Autodesk Inventor part; units mm, degrees
ref_plane "YZ Plane" through (0, 0, 0) normal (1, 0, 0) x (0, 1, 0)
ref_plane "XZ Plane" through (0, 0, 0) normal (0, 1, 0) x (-1, 0, 0)
ref_plane "XY Plane" through (0, 0, 0) normal (0, 0, 1) x (1, 0, 0)
sketch "Sketch1" plane through (0, 0, 0) normal (0, 0, 1) x (1, 0, 0)
  line L0 (-30, 40) -> (0, 40)
  line L1 (-36.1318, 34) -> (13.8682, 34) construction
  arc A0 (0, 30) -> (0, 38) centre (0, 34) ccw
  arc A1 (-30, 30) -> (-30, 38) centre (-30, 34) ccw
  line L2 (-30, 30) -> (0, 30) construction
  line L3 (-30, 0) -> (-30, -4.5) construction
  line L4 (-30, -4.5) -> (0, -4.5) construction
  line L5 (0, -4.5) -> (0, 0) construction
  circle A2 centre (-30, -4.5) radius 4 construction
  circle A3 centre (0, -4.5) radius 4 construction
  line L6 (-30, 0) -> (-30, 30)
  line L7 (-30, 38) -> (-30, 40)
  line L8 (0, 40) -> (0, 38)
  line L9 (0, 30) -> (0, 0)
  line L10 (-30, 0.0688) -> (-30, -0.5)
  line L11 (-30, -0.5) -> (-26, -4.5)
  line L12 (0, 0) -> (0, -0.5)
  line L13 (0, -0.5) -> (4, -4.5)
  line L14 (4, -4.5) -> (0, -8.5)
  line L15 (-26, -4.5) -> (-30, -8.5)
  line L16 (-30, -8.5) -> (-30, -10.5)
  line L17 (-30, -10.5) -> (0, -10.5)
  line L18 (0, -10.5) -> (0, -8.5)
  line L19 (0, 0) -> (-0.5, 0)
  dimension "d0" = 30
  dimension "d1" = 40
  dimension "d2" = 50
  dimension "d3" = 6
  dimension "d4" = 8
  dimension "d5" = 8
  dimension "d6" = 4.5
  dimension "d7" = 8
  dimension "d8" = 8
  dimension "d9" = 2
extrude "Extrusion1" add sketch "Sketch1" along normal blind 3
sketch "Sketch2" plane through (0, 0, 3) normal (0, 0, 1) x (1, 0, 0)
  line L0 (-30, -10.5) -> (0, -10.5) construction
  line L1 (0, -0.5) -> (0, 30) construction
  line L2 (0, 40) -> (-30, 40) construction
  line L3 (-15, 40) -> (-15, -10.5) construction
  line L4 (-15, 40) -> (-15, 36.5) construction
  line L5 (-15, 36.5) -> (-8.9843, 36.5) construction
  line L6 (-17.7725, 36.2895) -> (-9.6231, 36.2895) construction
  line L7 (-9.6231, 36.2895) -> (-9.6231, 27.3992) construction
  line L8 (-9.6231, 27.3992) -> (-17.7725, 27.3992) construction
  line L9 (-17.7725, 27.3992) -> (-17.7725, 36.2895) construction
  line L10 (-15, -10.5) -> (-15, 26) construction
  line L11 (-15, 26) -> (0, 26) construction
  line L12 (-5.7398, 26) -> (-28, 26)
  line L13 (-28, 26) -> (-28, 24)
  line L14 (-28, 24) -> (-5.7398, 24)
  line L15 (-5.7398, 24) -> (-5.7398, 26)
  line L16 (-28, 25) -> (0, 25) construction
  line L17 (-5.7398, 26) -> (-5.7398, 27.5)
  line L18 (-5.7398, 27.5) -> (-1.4096, 25)
  line L19 (-5.7398, 24) -> (-5.7398, 22.5)
  line L20 (-5.7398, 22.5) -> (-1.4096, 25)
  spline S0 degree 2 poles (-14.5989, 29.9621) (-15.2464, 29.9621) (-16.3191, 30.3575) (-16.7047, 30.7579) knots 0 0 0 1 2 2 2
  spline S1 degree 2 poles (-16.7047, 30.7579) (-17.0903, 31.1633) (-17.5006, 32.3596) (-17.5006, 33.1357) knots 0 0 0 1 2 2 2
  spline S2 degree 2 poles (-17.5006, 33.1357) (-17.5006, 33.8722) (-17.0853, 35.0388) (-16.6998, 35.4541) knots 0 0 0 1 2 2 2
  spline S3 degree 2 poles (-16.6998, 35.4541) (-16.329, 35.8545) (-15.2415, 36.2895) (-14.5939, 36.2895) knots 0 0 0 1 2 2 2
  spline S4 degree 2 poles (-14.5939, 36.2895) (-14.2825, 36.2895) (-13.719, 36.2005) (-13.4619, 36.1214) knots 0 0 0 1 2 2 2
  spline S5 degree 2 poles (-13.4619, 36.1214) (-13.2543, 36.0621) (-12.7501, 35.8446) (-12.5969, 35.7655) knots 0 0 0 1 2 2 2
  line L21 (-12.5969, 35.7655) -> (-12.5969, 34.7867)
  line L22 (-12.5969, 34.7867) -> (-12.6661, 34.7867)
  spline S6 degree 2 poles (-12.6661, 34.7867) (-12.8193, 34.9202) (-13.1406, 35.1624) (-13.4372, 35.3008) knots 0 0 0 1 2 2 2
  spline S7 degree 2 poles (-13.4372, 35.3008) (-13.6844, 35.4244) (-14.3221, 35.5875) (-14.6879, 35.5875) knots 0 0 0 1 2 2 2
  spline S8 degree 2 poles (-14.6879, 35.5875) (-15.5678, 35.5875) (-16.6553, 34.2627) (-16.6553, 33.1604) knots 0 0 0 1 2 2 2
  spline S9 degree 2 poles (-16.6553, 33.1604) (-16.6553, 32.5474) (-16.3686, 31.628) (-16.0967, 31.3116) knots 0 0 0 1 2 2 2
  spline S10 degree 2 poles (-16.0967, 31.3116) (-15.8347, 30.9952) (-15.0932, 30.664) (-14.6285, 30.664) knots 0 0 0 1 2 2 2
  spline S11 degree 2 poles (-14.6285, 30.664) (-14.2875, 30.664) (-13.6053, 30.7629) (-13.3729, 30.8618) knots 0 0 0 1 2 2 2
  line L23 (-13.3729, 30.8618) -> (-13.3729, 32.4387)
  line L24 (-13.3729, 32.4387) -> (-14.7867, 32.4387)
  line L25 (-14.7867, 32.4387) -> (-14.7867, 33.1505)
  line L26 (-14.7867, 33.1505) -> (-12.5721, 33.1505)
  line L27 (-12.5721, 33.1505) -> (-12.5721, 30.4861)
  spline S12 degree 2 poles (-12.5721, 30.4861) (-12.7254, 30.4169) (-13.2494, 30.2043) (-13.4718, 30.14) knots 0 0 0 1 2 2 2
  spline S13 degree 2 poles (-13.4718, 30.14) (-13.7734, 30.0511) (-14.2578, 29.9621) (-14.5989, 29.9621) knots 0 0 0 1 2 2 2
  point P0 (0, 0)
  dimension "d12" = 3.5
  dimension "d13" = 36.5
  dimension "d14" = 2
  dimension "d15" = 1.5
  dimension "d16" = 5
  dimension "d17" = 1.5
  dimension "d58" = 14
extrude "Extrusion2" cut sketch "Sketch2" against normal blind 1
sketch "Sketch5" plane through (0, 0, 0) normal (0, 0, -1) x (-1, 0, 0)
  line L0 (30, 30) -> (30, -0.5) construction
  arc A0 (30, 38) -> (30, 30) centre (30, 34) ccw construction
  line L1 (30, 40) -> (30, 38) construction
  line L2 (0, 40) -> (30, 40) construction
  line L3 (0, 38) -> (0, 40) construction
  arc A1 (0, 38) -> (0, 30) centre (0, 34) ccw construction
  line L4 (0, -0.5) -> (0, 30) construction
  line L5 (-4, -4.5) -> (0, -0.5) construction
  line L6 (0, -8.5) -> (-4, -4.5) construction
  line L7 (0, -10.5) -> (0, -8.5) construction
  line L8 (30, -10.5) -> (0, -10.5) construction
  line L9 (30, -8.5) -> (30, -10.5) construction
  line L10 (26, -4.5) -> (30, -8.5) construction
  line L11 (30, -0.5) -> (26, -4.5) construction
  point P0 (0, 0)
sketch "Sketch6" plane through (0, 0, 0) normal (0, 0, -1) x (-1, 0, 0)
  line L0 (30, 30) -> (30, -0.5) construction
  line L1 (0, 40) -> (30, 40) construction
  line L2 (30, -10.5) -> (0, -10.5) construction
  line L3 (17.9728, -6.9957) -> (10.1851, -6.9957) construction
  line L4 (10.1851, -6.9957) -> (10.1851, 2.1518) construction
  line L5 (10.1851, 2.1518) -> (17.9728, 2.1518) construction
  line L6 (17.9728, 2.1518) -> (17.9728, -6.9957) construction
  line L7 (15, -10.5) -> (15, 40) construction
  line L8 (15, -10.5) -> (15, -7) construction
  line L9 (15, -7) -> (11.2598, -7) construction
  line L10 (16.564, 40) -> (16.564, 4) construction
  line L11 (16.564, 4) -> (24.4907, 4) construction
  line L12 (30, 5.5) -> (28, 5.5) construction
  line L13 (28, 5.5) -> (6.5, 5.5)
  line L14 (6.5, 5.5) -> (6.5, 3.5)
  line L15 (6.5, 3.5) -> (28, 3.5)
  line L16 (28, 3.5) -> (28, 5.5)
  line L17 (6.5, 3.5) -> (6.5, 2)
  line L18 (6.5, 2) -> (2.1699, 4.5)
  line L19 (6.5, 5.5) -> (6.5, 7)
  line L20 (6.5, 7) -> (2.1699, 4.5)
  line L21 (5.7398, 24) -> (28, 24) construction
  line L22 (28, 26) -> (5.7398, 26) construction
  line L23 (1.1699, 23) -> (6.1699, 23)
  line L24 (6.1699, 23) -> (6.1699, 25)
  line L25 (6.1699, 25) -> (1.1699, 25)
  line L26 (1.1699, 25) -> (1.1699, 23)
  line L27 (7.1699, 23) -> (12.1699, 23)
  line L28 (12.1699, 25) -> (7.1699, 25)
  line L29 (12.1699, 23) -> (12.1699, 25)
  line L30 (7.1699, 25) -> (7.1699, 23)
  line L31 (13.1699, 23) -> (18.1699, 23)
  line L32 (18.1699, 25) -> (13.1699, 25)
  line L33 (18.1699, 23) -> (18.1699, 25)
  line L34 (13.1699, 25) -> (13.1699, 23)
  line L35 (19.1699, 23) -> (24.1699, 23)
  line L36 (24.1699, 25) -> (19.1699, 25)
  line L37 (24.1699, 23) -> (24.1699, 25)
  line L38 (19.1699, 25) -> (19.1699, 23)
  line L39 (24.1699, 23) -> (24.1699, 21.5)
  line L40 (24.1699, 21.5) -> (28.635, 23.75)
  line L41 (24.1699, 25) -> (24.1699, 26.5)
  line L42 (24.1699, 26.5) -> (28.635, 23.75)
  line L43 (0, -0.5) -> (0, 30) construction
  line L44 (28, 4.5) -> (0, 4.5) construction
  spline S0 degree 2 poles (14.7992, -0.6683) (15.4468, -0.6683) (16.5195, -1.0638) (16.9051, -1.4642) knots 0 0 0 1 2 2 2
  spline S1 degree 2 poles (16.9051, -1.4642) (17.2906, -1.8695) (17.7009, -3.0658) (17.7009, -3.8419) knots 0 0 0 1 2 2 2
  spline S2 degree 2 poles (17.7009, -3.8419) (17.7009, -4.5784) (17.2857, -5.745) (16.9001, -6.1603) knots 0 0 0 1 2 2 2
  spline S3 degree 2 poles (16.9001, -6.1603) (16.5294, -6.5607) (15.4419, -6.9957) (14.7943, -6.9957) knots 0 0 0 1 2 2 2
  spline S4 degree 2 poles (14.7943, -6.9957) (14.4829, -6.9957) (13.9193, -6.9067) (13.6623, -6.8276) knots 0 0 0 1 2 2 2
  spline S5 degree 2 poles (13.6623, -6.8276) (13.4547, -6.7683) (12.9505, -6.5508) (12.7972, -6.4717) knots 0 0 0 1 2 2 2
  line L45 (12.7972, -6.4717) -> (12.7972, -5.4929)
  line L46 (12.7972, -5.4929) -> (12.8664, -5.4929)
  spline S6 degree 2 poles (12.8664, -5.4929) (13.0197, -5.6264) (13.341, -5.8686) (13.6376, -6.007) knots 0 0 0 1 2 2 2
  spline S7 degree 2 poles (13.6376, -6.007) (13.8847, -6.1306) (14.5224, -6.2937) (14.8882, -6.2937) knots 0 0 0 1 2 2 2
  spline S8 degree 2 poles (14.8882, -6.2937) (15.7681, -6.2937) (16.8556, -4.9689) (16.8556, -3.8666) knots 0 0 0 1 2 2 2
  spline S9 degree 2 poles (16.8556, -3.8666) (16.8556, -3.2536) (16.5689, -2.3342) (16.2971, -2.0178) knots 0 0 0 1 2 2 2
  spline S10 degree 2 poles (16.2971, -2.0178) (16.0351, -1.7014) (15.2936, -1.3702) (14.8289, -1.3702) knots 0 0 0 1 2 2 2
  spline S11 degree 2 poles (14.8289, -1.3702) (14.4878, -1.3702) (13.8056, -1.4691) (13.5733, -1.568) knots 0 0 0 1 2 2 2
  line L47 (13.5733, -1.568) -> (13.5733, -3.1449)
  line L48 (13.5733, -3.1449) -> (14.9871, -3.1449)
  line L49 (14.9871, -3.1449) -> (14.9871, -3.8567)
  line L50 (14.9871, -3.8567) -> (12.7725, -3.8567)
  line L51 (12.7725, -3.8567) -> (12.7725, -1.1923)
  spline S12 degree 2 poles (12.7725, -1.1923) (12.9257, -1.1231) (13.4497, -0.9105) (13.6722, -0.8462) knots 0 0 0 1 2 2 2
  spline S13 degree 2 poles (13.6722, -0.8462) (13.9737, -0.7573) (14.4582, -0.6683) (14.7992, -0.6683) knots 0 0 0 1 2 2 2
  point P0 (0, 0)
  dimension "d36" = 3.5
  dimension "d37" = 36
  dimension "d38" = 2
  dimension "d39" = 1.5
  dimension "d40" = 5
  dimension "d41" = 1.5
  dimension "d42" = 5
  dimension "d43" = 2
  dimension "d46" = 6
  dimension "d51" = 1.5
  dimension "d52" = 5
  dimension "d53" = 1.5
  dimension "d56" = 18.5
  dimension "d57" = 14
extrude "Extrusion4" cut sketch "Sketch6" against normal blind 1
properties part number "MS_G[202] text"
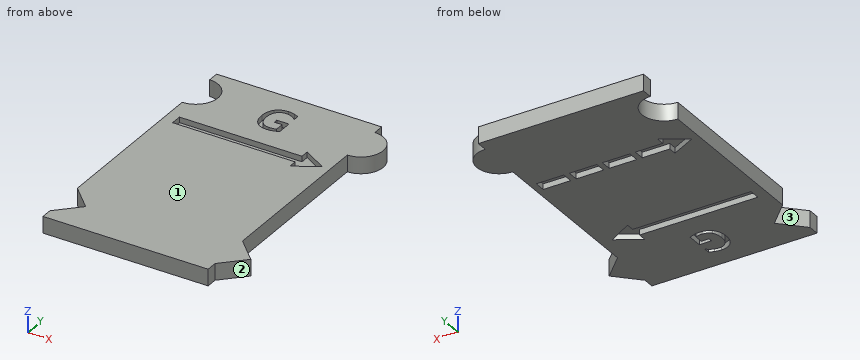
Part model, mm, in its own coordinate system. Face numbers are marked on the shaded views. Give positions to 0.01 mm unless a question says otherwise; leave off trailing zeros. Order: outer loops, then holes, each group sorted by start corner. A loop starts at its lowest first (then second) coordinate and runs counter-clockwise, first axis right, second up. Notation, with made-up numbers: (26.25, 69) - (71.25, 69) arc R27 cw to (71.25, 88) - close; hole circle Ø7 at (-25.5, -33.75). An arc over 180 degrees is marked (long way). Use a Markdown table: item, result.
1) Saw through at B-B on y = 19. List the corners of the cut face in (x, z).
Checked values:
| item | result |
|---|---|
| outline | (-30, 0) - (0, 0) - (0, 3) - (-30, 3) - close |
2) Probe L1, parallel to Y at x = -10.5, z = 0.25; L2, parallel to Y at x = -18.5, z = 0.4; L3, parallel to Y at x = -2, z = 0.8. List the from-to ranges inside material, lowest first. Write a range as from..to.
Checked values:
| item | result |
|---|---|
| L1 | -10.5..3.5, 5.5..23, 25..40 |
| L2 | -10.5..3.5, 5.5..40 |
| L3 | -10.5..23, 25..40 |
3) Flat gauge pins, fed straight in: P1, Ø0.6, axis at y = -10, z = 1.5, coming from the +X side; P2, Ø1.1, axis at y = -2, z = 0.5, coming from the -X side. Where does each tip first touch, or does it go through?
Checked values:
| item | result |
|---|---|
| P1 | x = 0 |
| P2 | x = -29.05 |
4) Saw through at A-A on x = -8. List the corners of the cut face in (y, z).
Checked values:
| item | result |
|---|---|
| outline | (-10.5, 0) - (3.5, 0) - (3.5, 1) - (5.5, 1) - (5.5, 0) - (23, 0) - (23, 1) - (25, 1) - (25, 0) - (40, 0) - (40, 3) - (26, 3) - (26, 2) - (24, 2) - (24, 3) - (-10.5, 3) - close |
5) Two-plate mould, pull along Y, no slides. Class the marked faces 1, 2 and 3: +Y half, -Y half, draft (parallel to the pull), parting line (faces both ways), or undercut.
Checked values:
| item | result |
|---|---|
| face 1 | draft |
| face 2 | -Y half |
| face 3 | undercut |
